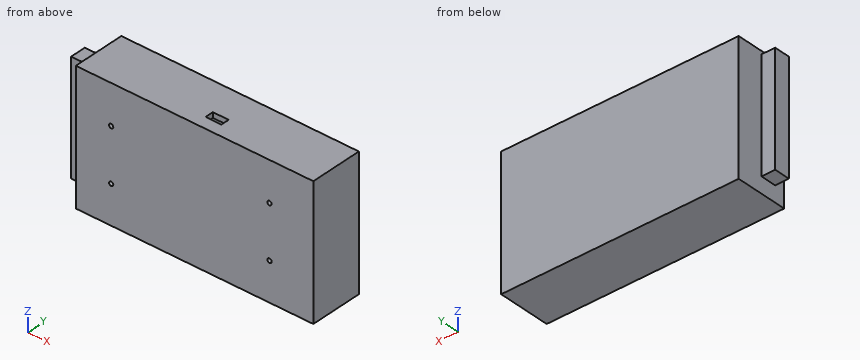
from build123d import *

# Parameters (mm, degrees)
SKETCH1_W           = 225
SKETCH1_H           = 124
BOSS_EXTRUDE1_DEPTH = 50
SKETCH3_R           = 2
CUT_EXTRUDE2_DEPTH  = 5
SKETCH4_W           = 15
SKETCH4_H           = 8
CUT_EXTRUDE3_DEPTH  = 5
SKETCH5_W           = 106
SKETCH5_H           = 15
BOSS_EXTRUDE2_DEPTH = 13


with BuildPart() as part:
    # Sketch1 → Boss-Extrude1 (new body)
    with BuildSketch(Plane(origin=(0, 0, 0), x_dir=(1, 0, 0), z_dir=(0, 1, 0))):
        Rectangle(SKETCH1_W, SKETCH1_H)
    extrude(amount=BOSS_EXTRUDE1_DEPTH)

    # Sketch3 → Cut-Extrude2 (cut)
    with BuildSketch(Plane.XZ):
        with Locations(Location((-79, -25.5, 0), (0, 0, 270))):  # turned: the seam where the file's is
            Circle(SKETCH3_R)
        with Locations(Location((-79, 24.5, 0), (0, 0, 270))):  # turned: the seam where the file's is
            Circle(SKETCH3_R)
        with Locations(Location((71, -25.5, 0), (0, 0, 270))):  # turned: the seam where the file's is
            Circle(SKETCH3_R)
        with Locations(Location((71, 24.5, 0), (0, 0, 270))):  # turned: the seam where the file's is
            Circle(SKETCH3_R)
    extrude(amount=-CUT_EXTRUDE2_DEPTH, mode=Mode.SUBTRACT)

    # Sketch4 → Cut-Extrude3 (cut)
    with BuildSketch(Plane.XY.offset(62)):
        with Locations((8, 15.5)):
            Rectangle(SKETCH4_W, SKETCH4_H)
    extrude(amount=-CUT_EXTRUDE3_DEPTH, mode=Mode.SUBTRACT)

    # Sketch5 → Boss-Extrude2 (add)
    with BuildSketch(Plane.ZY.offset(112.5)):
        with Locations((6, 17.5)):
            Rectangle(SKETCH5_W, SKETCH5_H)
    extrude(amount=BOSS_EXTRUDE2_DEPTH)


solid = part.part
Part model, mm, in its own coordinate system. Give positions to 0.01 mm unless a question says otherwise; leave off trailing zeros. Write each loop counter-clockwise with the first axis right and the second up, starting at its lowest first coordinate (ties: lowest second). Pieces come first, ordered by that corner, then holes.
1) Probe L1, parallel to X at y = 1.7, z = 24.5; L2, parallel to X at y = 3, z = 24; L3, parallel to X at y = 38.5, z = 32. List the from-to ranges inside material, lowest first.
Resolved:
L1: x = -112.5 to -81, -77 to 69, 73 to 112.5
L2: x = -112.5 to -80.94, -77.06 to 69.06, 72.94 to 112.5
L3: x = -112.5 to 112.5
2) Cut at A-A on y = 46. Write the cut outline in (x, z), then the cut area to 3 significant figures.
Resolved:
outline: (-112.5, -62) - (112.5, -62) - (112.5, 62) - (-112.5, 62) - close
area: 27,900 mm2
3) Pin check, flat tips, straight feed: pin 1 (10.5 mm diameter, centred on x = -119, z = -15.5, fed in from +Y); pin 2 (10.5 mm diameter, centred on x = -118, y = 15, fed in from +Z); pin 3 (10 mm diameter, centred on y = 40, z = 25, fed in from -X). Stop position of each tip, or through.
Resolved:
pin 1: stops at y = 25
pin 2: stops at z = 59
pin 3: stops at x = -112.5
